Source: CAD feature listing. Evaluate the final solid. Frame: model axes, mm. A direction names the side the tool comes from. Round coordinates to 2 decimals unless told otherwise and drop trailing zeros. Order: outer loops, then holes, each group sorted by start corner. A loop starts at its lowest first (then second) coordinate and runs counter-clockwise, first axis right, second up. Notation, with made-up numbers: (-30, 70.25) - (-18, 70.25) arc R20 ccw to (-18, 79.25) - close; hole circle Ø3 at (69, 46.25). An arc over 180 degrees is marked (long way). Return JSON: item names as keys, results as strings. Group by question number.
1) Section A-A, the plane y = 32.5. Return loops of the section in (x, z), plus the area to 3 significant figures.
2) Section D-D, the plane z = 1.5. Return loops of the section in (x, y).
3) Ray query, line 1 (X direction, y = 1.6, z = 7) (3 decimals); line 2 (Y direction, x = -7.5, z = 7); line 3 (Y direction, x = 2.85, z = 7). Return the intervals inside material, ascending. Write a range as from..to.
4) Section C-C, the plane y = 23. Return loops of the section in (x, z), plus the area to 3 significant figures.
5) Mould query, pull axis Y, two halves, no side actions, for faces 5 (the flat face through (6, 31, 9)), 6 (the flat face through (-5, 37.5, 7)), 7 (the cylindrical face through (-5.563, 30.864, 7.215)), 8 (the flat face through (0, 15, 14)). Classes: pulls with the +Y half, pulls with the -Y half, needs draft (parallel to the pull), parting line crosses it, or undercut.
6) Access query for faces 1 (the flat face through (-13, 6, 7)), 2 (the flat face through (10, 22, 7)), 3 (the cylindrical face through (3.54, 34.73, 7.29)), 4 (the flat face through (-1, 33, 5)). Directions: +Z, -Z, +X, -X, +Y, -Y. A direction counts if a zero-diameter tool reaches every point of the face in a straight line with its end or side. Return the directions, or none.
7) Contact query for flat-ended pins moving along their axis: P1, Ø6.5, axis at y = 31, z = 8, coming from the +X side; P2, Ø3, axis at y = 8.5, z = 2.5, coming from the -X side; P3, Ø4.5, axis at x = -16, z = 7, coming from the +Y side; P4, Ø4, axis at y = 31.5, z = 8, coming from the +X side. Output: stop coordinate, or through.
8) Section B-B, the plane x = -16. Return loops of the section in (y, z) (3 decimals).
```python
from build123d import *

# Parameters (mm, degrees)
SALIENTE_EXTRUIR1_DEPTH = 14
CROQUIS16_W             = 1.65
CROQUIS16_H             = 20
CORTAR_EXTRUIR3_REACH   = 8
CROQUIS4_R              = 2.625
REDONDEO0_75MM_R        = 0.75
CHAFL_N0_5MM_SIZE       = 0.5
CORTAR_EXTRUIR5_REACH   = 33
CROQUIS24_R             = 2.25
CROQUIS23_R             = 4
CORTAR_EXTRUIR4_DEPTH   = 4


with BuildPart() as part:
    # Croquis1 → Saliente-Extruir1 (new body)
    with BuildSketch(Plane.XY):
        with BuildLine():
            Line((-21, 6), (-21, 0))
            Line((-21, 0), (21, 0))
            Line((21, 0), (21, 6))
            Line((21, 6), (10, 6))
            Line((10, 6), (10, 37.5))
            Line((10, 37.5), (1, 37.5))
            Line((1, 37.5), (1, 28.916079783))
            ThreePointArc((1, 28.916079783), (0, 17), (-1, 28.916079783))
            Line((-1, 28.916079783), (-1, 37.5))
            Line((-1, 37.5), (-10, 37.5))
            Line((-10, 37.5), (-10, 6))
            Line((-10, 6), (-21, 6))
        make_face()
    extrude(amount=SALIENTE_EXTRUIR1_DEPTH)

    # Croquis16 → Taladro roscado M43 (revolve, cut)
    with BuildSketch(Plane(origin=(-1, 32.5, 7), x_dir=(0, 0, -1), z_dir=(0, 1, 0))):
        with Locations((0.825, 10)):
            Rectangle(CROQUIS16_W, CROQUIS16_H)
    revolve(axis=Axis((5.35, 32.5, 7), (-1, 0, 0)), mode=Mode.SUBTRACT)

    # Croquis4 → Cortar-Extruir3 (cut, up to next)
    with BuildSketch(Plane(origin=(0, 6, 0), x_dir=(1, 0, 0), z_dir=(0, 1, 0)), mode=Mode.PRIVATE) as cortar_extruir3_sk1:
        with Locations((-16, -7)):
            Circle(CROQUIS4_R)
    cortar_extruir3_tool1 = extrude(cortar_extruir3_sk1.sketch, amount=-CORTAR_EXTRUIR3_REACH, mode=Mode.PRIVATE) & part.part
    add(cortar_extruir3_tool1.solids().sort_by_distance((-16, 6, 7))[0], mode=Mode.SUBTRACT)
    # Croquis4 → Cortar-Extruir3 (cut, up to next)
    with BuildSketch(Plane(origin=(0, 6, 0), x_dir=(1, 0, 0), z_dir=(0, 1, 0)), mode=Mode.PRIVATE) as cortar_extruir3_sk2:
        with Locations((16, -7)):
            Circle(CROQUIS4_R)
    cortar_extruir3_tool2 = extrude(cortar_extruir3_sk2.sketch, amount=-CORTAR_EXTRUIR3_REACH, mode=Mode.PRIVATE) & part.part
    add(cortar_extruir3_tool2.solids().sort_by_distance((16, 6, 7))[0], mode=Mode.SUBTRACT)

    # Redondeo0,75mm
    redondeo0_75mm_edges = [part.edges().sort_by_distance(p)[0] for p in [
        (10, 37.5, 7),
        (10, 6, 7),
        (21, 6, 7),
        (-21, 6, 7),
        (-10, 6, 7),
        (-10, 37.5, 7),
    ]]
    fillet(redondeo0_75mm_edges, radius=REDONDEO0_75MM_R)

    # Chaflán0,5mm
    chafl_n0_5mm_edges = [part.edges().sort_by_distance(p)[0] for p in [
        (1, 37.5, 7),
        (-1, 37.5, 7),
    ]]
    chamfer(chafl_n0_5mm_edges, length=CHAFL_N0_5MM_SIZE)

    # Croquis24 → Cortar-Extruir5 (cut, up to next)
    with BuildSketch(Plane(origin=(10, 0, 0), x_dir=(0, 0, -1), z_dir=(1, 0, 0)), mode=Mode.PRIVATE) as cortar_extruir5_sk1:
        with Locations((-7, 32.5)):
            Circle(CROQUIS24_R)
    cortar_extruir5_tool1 = extrude(cortar_extruir5_sk1.sketch, amount=-CORTAR_EXTRUIR5_REACH, mode=Mode.PRIVATE) & part.part
    add(cortar_extruir5_tool1.solids().sort_by_distance((10, 32.5, 7))[0], mode=Mode.SUBTRACT)

    # Croquis23 → Cortar-Extruir4 (cut)
    with BuildSketch(Plane.ZY.offset(-10)):
        with Locations((7, 32.5)):
            Circle(CROQUIS23_R)
    extrude(amount=CORTAR_EXTRUIR4_DEPTH, mode=Mode.SUBTRACT)


solid = part.part
```
Geometry check:
{
 "1": {"outline": "(-10, 0) - (-1, 0) - (-1, 5.35) - (-10, 5.35) - close; (-10, 8.65) - (-1, 8.65) - (-1, 14) - (-10, 14) - close; (1, 0) - (10, 0) - (10, 3) - (6, 3) - (6, 4.75) - (1, 4.75) - close; (1, 9.25) - (6, 9.25) - (6, 11) - (10, 11) - (10, 14) - (1, 14) - close", "area": "168 mm2"},
 "2": {"outline": "(-21, 0) - (21, 0) - (21, 5.25) arc R0.75 ccw to (20.25, 6) - (10.75, 6) arc R0.75 cw to (10, 6.75) - (10, 36.75) arc R0.75 ccw to (9.25, 37.5) - (1.5, 37.5) - (1, 37) - (1, 28.92) arc R6 cw (long way) to (-1, 28.92) - (-1, 37) - (-1.5, 37.5) - (-9.25, 37.5) arc R0.75 ccw to (-10, 36.75) - (-10, 6.75) arc R0.75 cw to (-10.75, 6) - (-20.25, 6) arc R0.75 ccw to (-21, 5.25) - close"},
 "3": {"line 1": "-21..-18.625, -13.375..13.375, 18.625..21", "line 2": "0..30.85, 34.15..37.5", "line 3": "0..17.72, 28.28..30.25, 34.75..37.5"},
 "4": {"outline": "(-10, 0) - (-6, 0) - (-6, 14) - (-10, 14) - close; (6, 0) - (10, 0) - (10, 14) - (6, 14) - close", "area": "112 mm2"},
 "5": {"face 5": "undercut", "face 6": "pulls with the +Y half", "face 7": "undercut", "face 8": "needs draft"},
 "6": {"face 1": "+Z, -Z, -X, +Y", "face 2": "+Z, -Z, +X, +Y", "face 3": "+X", "face 4": "+Z, -Z, +Y"},
 "7": {"P1": "x = 10", "P2": "x = -10", "P3": "through", "P4": "x = 6"},
 "8": {"outline": "(0, 0) - (6, 0) - (6, 4.375) - (0, 4.375) - close; (0, 9.625) - (6, 9.625) - (6, 14) - (0, 14) - close"}
}
